```python
from build123d import *

# Parameters (mm, degrees)
CHAMFER1_SIZE = 5.2


with BuildPart() as part:
    # Sketch1 → Revolve1 (revolve)
    with BuildSketch(Plane.XY):
        Polygon((-11.59722846, 17.3), (-4.79722846, 17.3), (-4.79722846, -15.5), (-21.99722846, -15.5), (-21.99722846, 0), (-18.49722846, 0), (-18.49722846, -8.6), (-11.59722846, -8.6), align=None)
    revolve(axis=Axis((17.60277154, 25.472027778, 0), (0, -1, 0)))

    # Chamfer1
    chamfer1_edges = [part.edges().sort_by_distance(p)[0] for p in [
        (57.20277154, -15.5, 0),
    ]]
    chamfer(chamfer1_edges, length=CHAMFER1_SIZE)


solid = part.part
```
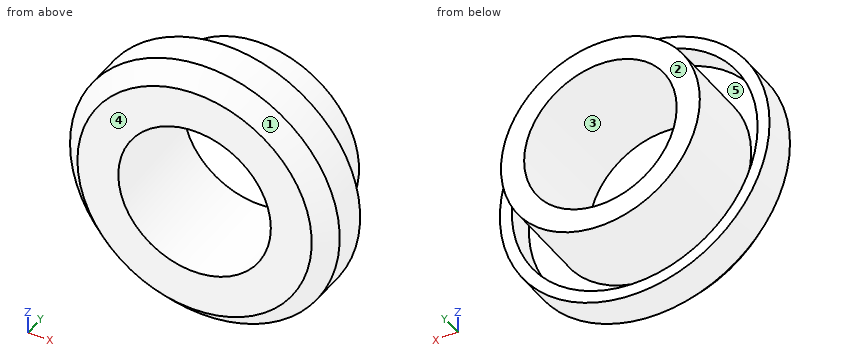
Can you work these out from the model? Positions are in its coordinate system, mm. Face numbers are marked on the shaded views. A direction names the side the tool comes from. Coordinates: 2 decimals unless noted, no trailing zeros. Loops run counter-clockwise (first coordinate to the right, second up) from the corner with the lowest first, then second, coordinate; pieces in that order, holes last. Notation, with made-up numbers: (-23, -6) - (12, -6) arc R13 cw to (12, 3) - close; hole circle Ø3 at (5.5, 0). An arc over 180 degrees is marked (long way). Use a Markdown table: item, result.
Item 1: I want a section at C-C on y = -11.5. Please give me the cut outline in (x, z).
Numbers:
| item | result |
|---|---|
| outline | circle Ø76.8 at (17.6, 0); hole circle Ø44.8 at (17.6, 0) |
Item 2: I want a section at A-A on z = 0. Please give me the cut outline in (x, y), and give its area (3 significant figures).
Numbers:
| item | result |
|---|---|
| outline | (-22, -10.3) - (-16.8, -15.5) - (-4.8, -15.5) - (-4.8, 17.3) - (-11.6, 17.3) - (-11.6, -8.6) - (-18.5, -8.6) - (-18.5, 0) - (-22, 0) - close; (40, -15.5) - (52, -15.5) - (57.2, -10.3) - (57.2, 0) - (53.7, 0) - (53.7, -8.6) - (46.8, -8.6) - (46.8, 17.3) - (40, 17.3) - close |
| area | 623 mm2 |
Item 3: Will these pins go through, and if not, where does the flat tip stop? pin 1 (6 mm diameter, centred on y = 0.5, z = -6.5, fed in from +X); pin 2 (2 mm diameter, centred on x = 1.5, z = -26, fed in from +Y); pin 3 (6 mm diameter, centred on x = 48, z = 28.5, fed in from -Y).
Numbers:
| item | result |
|---|---|
| pin 1 | stops at x = 57.04 |
| pin 2 | stops at y = -8.6 |
| pin 3 | stops at y = -11.23 |
Item 4: We'd pull the mould along Z, two halves only. Please class the marked faces 1, 2 and 3: released by +Z, released by -Z, zero draft, split by the parting line, or undercut.
Numbers:
| item | result |
|---|---|
| face 1 | split by the parting line |
| face 2 | zero draft |
| face 3 | undercut |
Item 5: I want a section at B-B on y = 15.5. Please give me the cut outline in (x, z).
Numbers:
| item | result |
|---|---|
| outline | circle Ø58.4 at (17.6, 0); hole circle Ø44.8 at (17.6, 0) |
Item 6: If I drill on probe 1 along X at (y, z) = (-3, 0); probe 2 along X at (y, z) = (8, 0); probe 3 along X at (y, z) = (-3, 8.5), over which ranges is the centre line in solid material (lowest first)? Write a range as from..to.
Numbers:
| item | result |
|---|---|
| probe 1 | x = -22..-18.5, -11.6..-4.8, 40..46.8, 53.7..57.2 |
| probe 2 | x = -11.6..-4.8, 40..46.8 |
| probe 3 | x = -21.07..-17.48, -10.33..-3.12, 38.33..45.54, 52.69..56.28 |
Item 7: For the marked faces 4 and 5, which set-ups out of +Z, -Z, +X, -X, +Y, -Y let a thin tool reach every point of the face, with its end or its side?
Numbers:
| item | result |
|---|---|
| face 4 | +Z, -Z, +X, -X, -Y |
| face 5 | +Y |
